For this review, take the finished solid that the model builds, in its own axes (mm). A direction names the side the tool comes from. Give positions to 0.01 mm unless a question says otherwise; leave off trailing zeros. Loops run counter-clockwise (first coordinate to the right, second up) from the corner with the lowest first, then second, coordinate; pieces in that order, holes last. Notation, with made-up numbers: (-3, -15) - (51, -15) arc R16 ccw to (51, 6) - close; hole circle Ø9 at (67.25, 49). An arc over 180 degrees is marked (long way). Answer in a Markdown table with one row per item.
```python
from build123d import *

# Parameters (mm, degrees)
F0_W      = 1700
F0_H      = 500
F1_DEPTH  = 25
F2_W      = 25
F2_H      = 500
F3_DEPTH  = 600
F6_W      = 1650
F6_H      = 25
F7_DEPTH  = 600
F8_W      = 25
F8_H      = 475
F9_DEPTH  = 600
F10_W     = 1165
F10_H     = 500
F11_DEPTH = 25
F12_R     = 10
F13_DEPTH = 510
F14_W     = 25
F14_H     = 150
F15_DEPTH = 1000
F16_W     = 25
F16_H     = 150
F17_DEPTH = 1000
F18_R     = 20
F19_DEPTH = 1650


with BuildPart() as f1:
    # F0 (on Top) → F1 (new body)
    with BuildSketch(Plane.XY):
        with Locations((850, 250)):
            Rectangle(F0_W, F0_H)
    extrude(amount=F1_DEPTH)

    # F2 (on face) → F3 (join)
    with BuildSketch(Plane.XY.offset(25)):
        with Locations((12.5, 250)):
            Rectangle(F2_W, F2_H)
    extrude(amount=F3_DEPTH)

    # F5: F1 across plane


with BuildPart() as f1_1:
    add(f1.part)
    add(f1.part.mirror(Plane.YZ.offset(850)))

    # F6 (on face) → F7 (join, through all)
    with BuildSketch(Plane.XY.offset(25)):
        with Locations((850, 487.5)):
            Rectangle(F6_W, F6_H)
    extrude(amount=F7_DEPTH)

    # F8 (on face) → F9 (join, through all)
    with BuildSketch(Plane.XY.offset(25)):
        with Locations((547.5, 237.5)):
            Rectangle(F8_W, F8_H)
    extrude(amount=F9_DEPTH)

    # F10 (on face) → F11 (join)
    with BuildSketch(Plane.XY.offset(625)):
        with Locations((1117.5, 250)):
            Rectangle(F10_W, F10_H)
    extrude(amount=-F11_DEPTH)

    # F12 (on face) → F13 (join, through all)
    with BuildSketch(Plane.YZ.offset(25)):
        with Locations((100, 605)):
            Circle(F12_R)
        with Locations((100, 205)):
            Circle(F12_R)
        with Locations((100, 405)):
            Circle(F12_R)
        with Locations((200, 605)):
            Circle(F12_R)
        with Locations((200, 405)):
            Circle(F12_R)
        with Locations((200, 205)):
            Circle(F12_R)
        with Locations((300, 605)):
            Circle(F12_R)
        with Locations((300, 405)):
            Circle(F12_R)
        with Locations((300, 205)):
            Circle(F12_R)
        with Locations((400, 605)):
            Circle(F12_R)
        with Locations((400, 405)):
            Circle(F12_R)
        with Locations((400, 205)):
            Circle(F12_R)
    extrude(amount=F13_DEPTH)

    # F14 (on face) → F15 (join)
    with BuildSketch(Plane.XY.offset(625)):
        with Locations((12.5, 250)):
            Rectangle(F14_W, F14_H)
    extrude(amount=F15_DEPTH)

    # F16 (on face) → F17 (join)
    with BuildSketch(Plane.XY.offset(625)):
        with Locations((1687.5, 250)):
            Rectangle(F16_W, F16_H)
    extrude(amount=F17_DEPTH)

    # F18 (on face) → F19 (join, through all)
    with BuildSketch(Plane.YZ.offset(25)):
        with Locations((250, 1585)):
            Circle(F18_R)
    extrude(amount=F19_DEPTH)


solid = f1_1.part
```
1. We need section A-A, the plane z = 732. Give the boundary of the cut face in (x, y).
Values:
| item | result |
|---|---|
| outline | (0, 175) - (25, 175) - (25, 325) - (0, 325) - close; (1675, 175) - (1700, 175) - (1700, 325) - (1675, 325) - close |
2. For faces 1 (the face through (1110, 241, 25)), 2 (the face through (838, 254, 0)), 3 (the face through (838.45, 247.4, 1604.83)), list the 3-axis set-ups (+Z, -Z, +X, -X, +Y, -Y) from which the entire face can be reached by the end or side of a thin tool; tool diameter is ignored.
Values:
| item | result |
|---|---|
| face 1 | -Y |
| face 2 | -Z, +X, -X, +Y, -Y |
| face 3 | none |
3. We need section D-D, the plane x = 1031. Give the boundary of the cut face in (y, z).
Values:
| item | result |
|---|---|
| outline | (0, 0) - (500, 0) - (500, 625) - (0, 625) - (0, 600) - (475, 600) - (475, 25) - (0, 25) - close; circle Ø40 at (250, 1585) |
4. We need section B-B, the plane x = 394.5. Count the separate pieces of the cut face and the enclosed holes in it, and give its area (3 significant figures).
Values:
| item | result |
|---|---|
| separate pieces | 14 |
| enclosed holes | 0 |
| area | 32,500 mm^2 |
5. We need section C-C, the plane y = 250. Give the boundary of the cut face in (x, z).
Values:
| item | result |
|---|---|
| outline | (0, 0) - (1700, 0) - (1700, 1625) - (1675, 1625) - (1675, 1605) - (25, 1605) - (25, 1625) - (0, 1625) - close; hole (25, 25) - (535, 25) - (535, 625) - (1675, 625) - (1675, 1565) - (25, 1565) - close; hole (560, 25) - (1675, 25) - (1675, 600) - (560, 600) - close |
6. Clearance check with flat-ended pins moving along their axes: pin 1 (7.5 mm diameter, centred on x = 18, z = 1099.5, fed in from +Y); pin 2 (6 mm diameter, centred on x = 1014.5, y = 309.5, fed in from +Z); pin 3 (12.5 mm diameter, centred on x = 1691, z = 921, fed in from -Y). State where each tip first meets the part, or that it passes through.
Values:
| item | result |
|---|---|
| pin 1 | stops at y = 325 |
| pin 2 | stops at z = 625 |
| pin 3 | stops at y = 175 |
7. Mouldability with a two-part tool opening along X and no side actions: class faces 4 (the face through (791, 0, 10)), 5 (the face through (276, 241, 25)), 6 (the face through (0, 247, 621)) as released by +X, released by -X, zero draft, split by the parting line, or undercut.
Values:
| item | result |
|---|---|
| face 4 | zero draft |
| face 5 | undercut |
| face 6 | released by -X |
8. Wall thickness on line 1 (X direction, y = 104, z = 574); line 2 (Z direction, x = 677, y = 471.5); line 3 (X direction, y = 269.5, z = 1470): over which ranges is each line inside the solid? List them lowest first. Write a range as [from, to].
Values:
| item | result |
|---|---|
| line 1 | x = [0, 25], [535, 560], [1675, 1700] |
| line 2 | z = [0, 25], [600, 625] |
| line 3 | x = [0, 25], [1675, 1700] |
